The model under review builds one solid part; all positions refer to its coordinate system, in mm. Face numbers are marked on the shaded views. A direction names the side the tool comes from. Round coordinates to 2 decimals unless told otherwise and drop trailing zeros. Order: outer loops, then holes, each group sorted by start corner. A loop starts at its lowest first (then second) coordinate and runs counter-clockwise, first axis right, second up. Notation, with made-up numbers: M -35,67 L -30,67 A25 ccw -30,79 Z; hole C 82.25,73.25 d9. An arc over 180 degrees is marked long. Answer as a JSON object with one key per item and string values. Group by question number.
1. Clearance check with flat-ended pins moving along their axes: P1, Ø11.5, axis at x = 34.15, z = -36.1, coming from the +Y side; P2, Ø3.5, axis at x = -33.5, y = -33.5, coming from the +Z side; P3, Ø3.5, axis at x = 33, y = -34.5, coming from the +Z side; P4, Ø2.5, axis at x = -32.5, y = 32.5, coming from the -Z side. State where each tip first meets the part, or that it passes through.
2. Mouldability with a two-part tool opening along X and no side actions: class the marked faces 3, 4, 5 and 6 as released by +X, released by -X, zero draft, split by the parting line, or undercut.
3. Add section B-B on y = 0. State the section outline as (x, z) points.
4. Add section A-A on z = -80. State the section outline as (x, y) points, and give its area (3 significant figures).
5. To check wall thickness, follow probe 1 along X at (y, z) = (9, -48); probe 2 along X at (y, z) = (-22.5, -49.1); probe 3 along Y at (x, z) = (34.2, -124.85). State the ranges of each line that lie inside material, in increasing order. Write a range as [from, to].
6. Machinability: for the marked faces 1 and 2, which of the approach directions +Z, -Z, +X, -X, +Y, -Y give a long, thin tool a straight path to every point of the face, cutting with its end or side? Answer none if there is none.
7. Add section C-C on z = -36.1. State the section outline as (x, y) points.
8. Add section D-D on y = 32.5. State the section outline as (x, z) points (3 decimals), and give its area (3 significant figures).
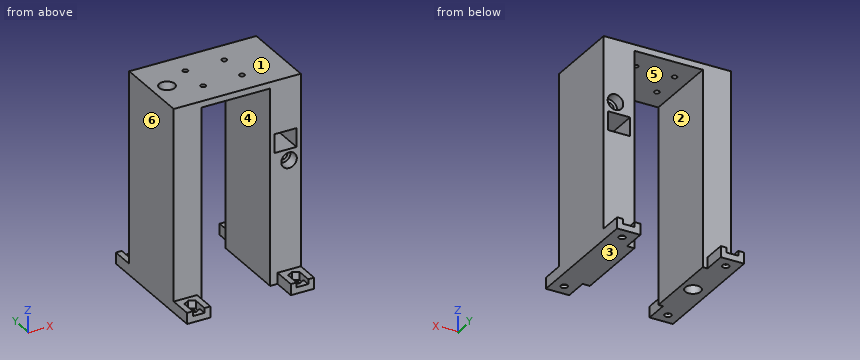
Autodesk Inventor part; units mm, degrees
ref_plane "Endfläche-ProbeHeadarme" through (0, 0, -126) normal (0, 0, 1) x (1, 0, 0)
ref_plane "Z-LowerBelt" through (0, 0, -49.1) normal (0, 0, 1) x (1, 0, 0)
ref_plane "X-Belts" through (26.75, 0, 0) normal (1, 0, 0) x (0, 1, 0)
sketch "S-ProbeHead-BaseSkizze" plane through (0, 0, 0) normal (0, 0, 1) x (1, 0, 0)
  line L0 (-40, 40) -> (40, 40)
  line L1 (40, 40) -> (40, -40)
  line L2 (40, -40) -> (-40, -40)
  line L3 (-40, -40) -> (-40, 40)
  line L4 (-40, 40) -> (40, -40) construction
  line L5 (40, 40) -> (-40, -40) construction
  line L6 (-56.34, 0) -> (58.04, 0) construction
  circle A0 centre (-30, 0) radius 5
  line L7 (0, 83.0683) -> (0, -88.0384) construction
  line L8 (-7.5, 58.6245) -> (-7.5, -60.8735) construction
  line L9 (-16, 21) -> (16, 21) construction
  line L10 (16, 21) -> (16, -21) construction
  line L11 (16, -21) -> (-16, -21) construction
  line L12 (-16, -21) -> (-16, 21) construction
  line L13 (-16, 21) -> (16, -21) construction
  line L14 (16, 21) -> (-16, -21) construction
  circle A1 centre (-12.5, -10) radius 1.65
  circle A2 centre (-12.5, 10) radius 1.65
  circle A3 centre (12.5, -10) radius 1.65
  circle A4 centre (12.5, 10) radius 1.65
  line L15 (-20, 57.6709) -> (-20, -63.5946)
  line L16 (7.5, 58.6245) -> (7.5, -60.8735) construction
  line L17 (20, 57.6709) -> (20, -63.5946)
  line L18 (41.7, 25) -> (-40, 25)
  line L19 (-40, 25) -> (-40, -25)
  line L20 (-40, -25) -> (41.7, -25)
  line L21 (41.7, -25) -> (41.7, 25)
  line L22 (22, 25) -> (22, -25)
  line L23 (-22, -25) -> (-22, 25)
  point P0 (0, 0)
  point P1 (41.7, 0)
  dimension "d1" = 80
  dimension "d2" = 80
  dimension "d4" = 10
  dimension "d6" = 30
  dimension "d20" = 7.5
  dimension "d21" = 32
  dimension "d22" = 42
  dimension "d23" = 3.3
  dimension "d24" = 10
  dimension "d25" = 12.5
  dimension "d26" = 20
  dimension "d27" = 50
  dimension "d30" = 20
  dimension "d31" = 21.7
  dimension "d32" = 2
  dimension "d37" = 2
extrude "BasePlate" add sketch "S-ProbeHead-BaseSkizze" along normal blind 4 contours L18 L23 L20 L3 | L18 L17 L20 L15 | L15 L20 L23 L18 | L18 L22 L20 L17 | L18 L21 L20 L1 | L1 L20 L22 L18
ref_plane "Endfläche-ProbeHeadarme" through (0, 0, -126) normal (0, 0, 1) x (1, 0, 0)
ref_plane "ProfilDownside" through (0, 0, -56) normal (0, 0, 1) x (1, 0, 0)
extrude "Arms" add sketch "S-ProbeHead-BaseSkizze" against normal up to surface (126 mm away) contours L18 L23 L20 L3 | L18 L21 L20 L1 | L1 L20 L22 L18
ref_plane "Z-UpperBelt" through (0, 0, -36.1) normal (0, 0, 1) x (1, 0, 0)
ref_plane "Z-LowerBelt" through (0, 0, -49.1) normal (0, 0, 1) x (1, 0, 0)
ref_plane "X-Belts" through (26.75, 0, 0) normal (1, 0, 0) x (0, 1, 0)
sketch "S-Tensioners" plane through (-40, -25, 4) normal (0, -1, 0) x (1, 0, 0)
  line L0 (64.75, -47.25) -> (78.95, -47.25)
  line L1 (78.95, -47.25) -> (78.95, -58.95)
  line L2 (78.95, -58.95) -> (64.75, -58.95)
  line L3 (64.75, -58.95) -> (64.75, -47.25)
  line L4 (64.75, -47.25) -> (78.95, -58.95) construction
  line L5 (78.95, -47.25) -> (64.75, -58.95) construction
  line L6 (71.85, -74) -> (71.85, 12.5724) construction
  line L7 (-16.34, -40.1) -> (98.04, -40.1) construction
  line L8 (-16.34, -53.1) -> (98.04, -53.1) construction
  circle A0 centre (74.15, -53.1) radius 2.9
  line L9 (64.75, -34.25) -> (78.95, -34.25)
  line L10 (78.95, -34.25) -> (78.95, -45.95)
  line L11 (78.95, -45.95) -> (64.75, -45.95)
  line L12 (64.75, -45.95) -> (64.75, -34.25)
  line L13 (64.75, -34.25) -> (78.95, -45.95) construction
  line L14 (78.95, -34.25) -> (64.75, -45.95) construction
  circle A1 centre (74.15, -40.1) radius 2.9
  circle A2 centre (74.15, -40.1) radius 5
  circle A3 centre (74.15, -53.1) radius 5
  line L15 (66.75, 41.0869) -> (66.75, -158.5145) construction
  line L16 (78.95, -34.25) -> (64.75, -34.25)
  line L17 (64.75, -34.25) -> (64.75, -33.95)
  line L18 (64.75, -33.95) -> (78.95, -33.95)
  line L19 (78.95, -33.95) -> (78.95, -34.25)
  line L20 (78.95, -58.95) -> (64.75, -58.95)
  line L21 (64.75, -58.95) -> (64.75, -59.25)
  line L22 (64.75, -59.25) -> (78.95, -59.25)
  line L23 (78.95, -59.25) -> (78.95, -58.95)
  point P0 (40, -4)
  point P1 (78.95, -40.1)
  point P2 (78.95, -53.1)
  dimension "d38" = 14.2
  dimension "d39" = 11.7
  dimension "d42" = 5.8
  dimension "d43" = 14.2
  dimension "d44" = 11.7
  dimension "d45" = 5.8
  dimension "d53" = 4.8
  dimension "d54" = 4.8
  dimension "d55" = 10
  dimension "d56" = 10
  dimension "d58" = 7.4
  dimension "d59" = 7.4
  dimension "d79" = 0.3
  dimension "d80" = 0.3
extrude "Ex-Tensioners1-Holes" cut sketch "S-Tensioners" against normal blind 50 contours A0 | A1
extrude "Ex-Tensioners2-SlideVolume" cut sketch "S-Tensioners" along normal blind 35 from surface at -50 contours L0 L1 A3 L2 L3 | L2 L23 L22 L21 | L1 A3 picked at (78.3167, -53.1)
extrude "Ex-Tensioners3-SlideVolume" cut sketch "S-Tensioners" against normal blind 35 contours L17 L18 L19 L9 | L9 L10 A2 L11 L12 | L10 A2 picked at (78.3167, -40.1)
extrude "Ex-Tensioners4-SrewHead" cut sketch "S-Tensioners" against normal blind 7 contours A3 L1 | L1 A3
extrude "Ex-Tensioners5-SrewHead" cut sketch "S-Tensioners" along normal blind 7 from surface at -50 contours A2 L10 | L10 A2
sketch "S-Anschraubpunkte-ProbeAntenna" plane through (0, 0, -126) normal (0, 0, 1) x (1, 0, 0)
  line L0 (-56.34, 0) -> (58.04, 0) construction
  line L1 (0, 74.3335) -> (0, -68.3114) construction
  line L2 (41.7, 25) -> (-40, 25)
  line L3 (41.7, -25) -> (41.7, 25)
  line L4 (-40, -25) -> (41.7, -25)
  line L5 (-40, 25) -> (-40, -25)
  line L6 (41.7, 25) -> (26.7, 25)
  line L7 (26.7, 25) -> (26.7, 40)
  line L8 (26.7, 40) -> (41.7, 40)
  line L9 (41.7, 40) -> (41.7, 25)
  line L10 (22, -25) -> (22, 25)
  line L11 (22, 25) -> (22, -25)
  line L12 (-22, 25) -> (-22, -25)
  line L13 (-22, -25) -> (-22, 25)
  line L14 (41.7, 32.5) -> (26.7, 32.5) construction
  line L15 (34.2, 40) -> (34.2, 25) construction
  circle A0 centre (34.2, 32.5) radius 2.15
  circle A1 centre (34.2, 32.5) radius 4 construction
  line L16 (0.85, 53.9557) -> (0.85, -47.9335) construction
  line L17 (-40, 25) -> (-25, 25)
  line L18 (-25, 25) -> (-25, 40)
  line L19 (-25, 40) -> (-40, 40)
  line L20 (-40, 40) -> (-40, 25)
  circle A2 centre (-32.5, 32.5) radius 2.15
  circle A3 centre (-32.5, 32.5) radius 4 construction
  line L21 (41.7, -25) -> (26.7, -25)
  line L22 (26.7, -25) -> (26.7, -40)
  line L23 (26.7, -40) -> (41.7, -40)
  line L24 (41.7, -40) -> (41.7, -25)
  circle A4 centre (34.2, -32.5) radius 2.15
  circle A5 centre (34.2, -32.5) radius 4 construction
  line L25 (-40, -40) -> (-40, -25)
  line L26 (-25, -40) -> (-40, -40)
  line L27 (-40, -25) -> (-25, -25)
  line L28 (-25, -25) -> (-25, -40)
  circle A6 centre (-32.5, -32.5) radius 4 construction
  circle A7 centre (-32.5, -32.5) radius 2.15
  line L29 (34.2, 28.1987) -> (30.475, 30.3494)
  line L30 (30.475, 30.3494) -> (30.475, 40)
  line L31 (30.475, 34.6506) -> (34.2, 36.8013)
  line L32 (34.2, 36.8013) -> (37.925, 34.6506)
  line L33 (37.925, 40) -> (37.925, 30.3494)
  line L34 (37.925, 30.3494) -> (34.2, 28.1987)
  line L35 (34.2, -28.1987) -> (30.475, -30.3494)
  line L36 (30.475, -30.3494) -> (30.475, -40)
  line L37 (30.475, -34.6506) -> (34.2, -36.8013)
  line L38 (34.2, -36.8013) -> (37.925, -34.6506)
  line L39 (37.925, -40) -> (37.925, -30.3494)
  line L40 (37.925, -30.3494) -> (34.2, -28.1987)
  line L41 (-32.5, 28.1987) -> (-28.775, 30.3494)
  line L42 (-28.775, 30.3494) -> (-28.775, 40)
  line L43 (-28.775, 34.6506) -> (-32.5, 36.8013)
  line L44 (-32.5, 36.8013) -> (-36.225, 34.6506)
  line L45 (-36.225, 40) -> (-36.225, 30.3494)
  line L46 (-36.225, 30.3494) -> (-32.5, 28.1987)
  line L47 (-36.225, -40) -> (-36.225, -30.3494)
  line L48 (-32.5, -36.8013) -> (-36.225, -34.6506)
  line L49 (-28.775, -34.6506) -> (-32.5, -36.8013)
  line L50 (-28.775, -30.3494) -> (-28.775, -40)
  line L51 (-32.5, -28.1987) -> (-28.775, -30.3494)
  line L52 (-36.225, -30.3494) -> (-32.5, -28.1987)
  point P0 (0, 0)
  dimension "d46" = 50
  dimension "d67" = 15
  dimension "d68" = 15
  dimension "d69" = 4.3
  dimension "d70" = 8
  dimension "d71" = 81.7
  dimension "d72" = 40.85
  dimension "d75" = 65
  dimension "d76" = 66.7
  dimension "d81" = 7.45
extrude "Ex-Anschraubpunkte-Eb1" add sketch "S-Anschraubpunkte-ProbeAntenna" along normal blind 2 contours L2 L7 L8 L30 L29 L34 L33 L9 | L24 L23 L39 L40 L35 L36 L22 L4 | L33 L32 L31 L30 L8 | L23 L36 L37 L38 L39 | L33 L34 L29 L30 L31 L32 | L2 L20 L19 L45 L46 L41 L42 L18 | L38 L37 L36 L35 L40 L39 | L28 L26 L50 L51 L52 L47 L25 L4 | L42 L43 L44 L45 L19 | L42 L41 L46 L45 L44 L43 | L26 L47 L48 L49 L50 | L49 L48 L47 L52 L51 L50
extrude "Ex-Anschraubpunkte-Eb2" add sketch "S-Anschraubpunkte-ProbeAntenna" along normal blind 2 from surface at 2 contours L2 L7 L8 L30 L29 L34 L33 L9 | L24 L23 L39 L40 L35 L36 L22 L4 | L33 L32 L31 L30 L8 | L23 L36 L37 L38 L39 | L2 L20 L19 L45 L46 L41 L42 L18 | L28 L26 L50 L51 L52 L47 L25 L4 | L42 L43 L44 L45 L19 | L26 L47 L48 L49 L50
extrude "Ex-Anschraubpunkte-Eb3" add sketch "S-Anschraubpunkte-ProbeAntenna" along normal blind 3.1 from surface at 4 contours L2 L7 L8 L30 L29 L34 L33 L9 | L24 L23 L39 L40 L35 L36 L22 L4 | L2 L20 L19 L45 L46 L41 L42 L18 | L28 L26 L50 L51 L52 L47 L25 L4
extrude "Ex-Anschraubpunkte-Eb4" [suppressed]
ref_plane "Anschraubpunkt-Spiegelebene" through (0.85, 53.9557, -126) normal (-1, 0, 0) x (0, -1, 0)
ref_plane "ProfilTopSide" through (0, 0, -16) normal (0, 0, 1) x (1, 0, 0)
equation "\"d43\" = d38"
equation "\"d44\" = d39"
equation "\"d45\" = d42"
equation "\"d53\" = d54"
equation "\"d55\" = d56"
equation "\"d58\" = d59"
equation "\"d80\" = d79"
equation "\"d72\" = 0.5 * d71"
properties part number "ProbeHead-BaseBody V3"
Recorded:
{
 "1": {"P1": "stops at y = 25", "P2": "stops at z = -124", "P3": "stops at z = -122", "P4": "passes through"},
 "2": {"face 3": "zero draft", "face 4": "undercut", "face 5": "undercut", "face 6": "released by -X"},
 "3": {"outline": "M -40,-126 L -35,-126 L -35,4 L -40,4 Z; M -25,-126 L -22,-126 L -22,0 L 22,0 L 22,-126 L 41.7,-126 L 41.7,4 L -25,4 Z; hole M 24.75,-55.25 L 38.95,-55.25 L 38.95,-43.25 L 24.75,-43.25 Z; hole M 24.75,-41.95 L 38.95,-41.95 L 38.95,-29.95 L 24.75,-29.95 Z"},
 "4": {"outline": "M -40,-25 L -22,-25 L -22,25 L -40,25 Z; M 22,-25 L 41.7,-25 L 41.7,25 L 22,25 Z; hole C -30,0 d10", "area": "1,810 mm²"},
 "5": {"probe 1": "x = [-40, -22], [22, 24.75], [38.95, 41.7]", "probe 2": "x = [-40, -22], [22, 29.15], [39.15, 41.7]", "probe 3": "y = [-40, -34.65], [-30.35, 30.35], [34.65, 40]"},
 "6": {"face 1": "+Z, +X, -X, +Y, -Y", "face 2": "-Z, +Y, -Y"},
 "7": {"outline": "M -40,-25 L -22,-25 L -22,25 L -40,25 Z; M 22,-25 L 24.75,-25 L 24.75,10 L 31.25,10 L 31.25,18 L 29.15,18 L 29.15,25 L 22,25 Z; M 37.05,10 L 38.95,10 L 38.95,-25 L 41.7,-25 L 41.7,25 L 39.15,25 L 39.15,18 L 37.05,18 Z; hole C -30,0 d10"},
 "8": {"outline": "M -40,-126 L -34.65,-126 L -34.65,-124 L -36.225,-124 L -36.225,-118.9 L -40,-118.9 Z; M -30.35,-126 L -25,-126 L -25,-118.9 L -28.775,-118.9 L -28.775,-124 L -30.35,-124 Z; M 26.7,-126 L 32.05,-126 L 32.05,-124 L 30.475,-124 L 30.475,-118.9 L 26.7,-118.9 Z; M 36.35,-126 L 41.7,-126 L 41.7,-118.9 L 37.925,-118.9 L 37.925,-124 L 36.35,-124 Z", "area": "120 mm²"}
}
